Design review of the part built by this model. Coordinates are the model's own, in mm. A direction names the side the tool comes from. Coordinates: 2 decimals unless noted, no trailing zeros. Order: outer loops, then holes, each group sorted by start corner. A loop starts at its lowest first (then second) coordinate and runs counter-clockwise, first axis right, second up. Notation, with made-up numbers: (67.25, 60.25) - (106.25, 60.25) arc R30 ccw to (106.25, 96.25) - close; hole circle Ø5 at (-16.5, 39). An arc over 180 degrees is marked (long way). Write each question's results on one line, items separated by ' | '. Start each with the question number.
```python
from build123d import *

# Parameters (mm, degrees)
ESQUISSE1_R                  = 12.5
BOSS_EXTRU_1_DEPTH           = 34.6
BOSS_EXTRU_2_START           = -34.6
BOSS_EXTRU_2_DEPTH           = 34.6
R_P_TITION_CIRCULAIRE1_COUNT = 12
ESQUISSE5_R                  = 7.5
ENL_V_MAT_EXTRU_2_DEPTH      = 5
ESQUISSE6_R                  = 6
ENL_V_MAT_EXTRU_3_DEPTH      = 24.6
ENL_V_START                  = -5
ESQUISSE7_R                  = 7.5
ENL_V_MAT_EXTRU_4_DEPTH      = 5


with BuildPart() as part:
    # Esquisse1 → Boss.-Extru.1 (new body)
    with BuildSketch(Plane.XY):
        Circle(ESQUISSE1_R)
    extrude(amount=BOSS_EXTRU_1_DEPTH)

    # Esquisse3 → Boss.-Extru.2 (add)
    with BuildSketch(Plane.XY.offset(34.6).offset(BOSS_EXTRU_2_START)):
        with BuildLine():
            Line((-1, 17.810368556), (-2.169061089, 12.310368556))
            ThreePointArc((-2.169061089, 12.310368556), (0, 12.5), (2.169061089, 12.310368556))
            Line((2.169061089, 12.310368556), (1, 17.810368556))
            Line((1, 17.810368556), (-1, 17.810368556))
        make_face()
    boss_extru_2 = extrude(amount=BOSS_EXTRU_2_DEPTH)

    # R_p_tition circulaire1: Boss.-Extru.2 ×12 about axis
    r_p_tition_circulaire1_axis = Axis((0, 0, 0), (0, 0, 1))
    for i in range(1, R_P_TITION_CIRCULAIRE1_COUNT):
        add(boss_extru_2.rotate(r_p_tition_circulaire1_axis, i * 360 / R_P_TITION_CIRCULAIRE1_COUNT))

    # Esquisse5 → Enl_v. mat.-Extru.2 (cut)
    with BuildSketch(Plane.XY.offset(34.6)):
        Circle(ESQUISSE5_R)
    extrude(amount=-ENL_V_MAT_EXTRU_2_DEPTH, mode=Mode.SUBTRACT)

    # Esquisse6 → Enl_v. mat.-Extru.3 (cut)
    with BuildSketch(Plane.XY.offset(29.6)):
        Circle(ESQUISSE6_R)
    extrude(amount=-ENL_V_MAT_EXTRU_3_DEPTH, mode=Mode.SUBTRACT)

    # Esquisse7 → Enl_v. mat.-Extru.4 (cut)
    with BuildSketch(Plane(origin=(0, 0, 0), x_dir=(-1, 0, 0), z_dir=(0, 0, -1)).offset(ENL_V_START)):
        with Locations(Location((0, 0, 0), (0, 0, 180))):
            Circle(ESQUISSE7_R)
    extrude(amount=ENL_V_MAT_EXTRU_4_DEPTH, mode=Mode.SUBTRACT)


solid = part.part
```
(1) Take a section at D-D (x = 10.5). State the section outline as (y, z) points, plus the area to 3 significant figures.
(2) Take a section at C-C (x = -13). State the section outline as (y, z) points, plus the area to 3 significant figures.
(3) Tool access review of faces 1 (the face through (6.132, -13.806, 17.058)), 2 (the face through (-15.022, 1.593, 17.058)), 3 (the face through (3.25, 12.07, 17.06)), 4 (the face through (-8.85, -8.83, 17.06)): name each direction out of +Z, -Z, +X, -X, +Y, -Y from which nothing blocks a thin tool from reaching the whole face with its end or side.
(4) Clearance check with flat-ended pins moving along their axes: pin 1 (9 mm diameter, centred on x = 0, y = 0, fed in from -Z); pin 2 (1 mm diameter, centred on x = 8.5, z = 26.5, fed in from +Y); pin 3 (10 mm diameter, centred on y = 8.5, z = 9.5, fed in from +X); pin 4 (2 mm diameter, centred on x = 4, z = 14.5, fed in from -Y). State where each tip first meets the part, or that it passes through.
(5) Take a section at A-A (y = 0). State the section outline as (x, z) points.
(6) To check wall thickness, follow line 1 along Y through (x, z) = (0, 4); line 2 along Y through (x, z) = (14, 18); line 3 along Y through (x, z) = (0, 16.25). State the ranges of each line that lie inside material, in increasing order. Write a range as [from, to].
(7) Mouldability with a two-part tool opening along Y and no side actions: class faces 5 (the face through (15.431, 8.893, 17.058)), 6 (the face through (-17.81, 0, 17)), 7 (the face through (12.07, -3.25, 17.06)) as +Y half, -Y half, draft (parallel to the pull), parting line (faces both ways), or undercut.
Worked out:
1) outline: (-8.33, 0) - (8.33, 0) - (8.33, 34.6) - (-8.33, 34.6) - close | area: 577 mm^2
2) outline: (-9.15, 0) - (-5.41, 0) - (-5.41, 34.6) - (-9.15, 34.6) - close; (-2.02, 0) - (2.02, 0) - (2.02, 34.6) - (-2.02, 34.6) - close; (5.41, 0) - (9.15, 0) - (9.15, 34.6) - (5.41, 34.6) - close | area: 399 mm^2
3) face 1: +Z, -Z, -Y | face 2: +Z, -Z, -X | face 3: +Z, -Z, +Y | face 4: +Z, -Z
4) pin 1: through | pin 2: y = 15.92 | pin 3: x = 15.92 | pin 4: y = -12.55
5) outline: (-17.81, 0) - (-7.5, 0) - (-7.5, 5) - (-6, 5) - (-6, 29.6) - (-7.5, 29.6) - (-7.5, 34.6) - (-17.81, 34.6) - close; (6, 5) - (7.5, 5) - (7.5, 0) - (17.81, 0) - (17.81, 34.6) - (7.5, 34.6) - (7.5, 29.6) - (6, 29.6) - close
6) line 1: [-17.81, -7.5], [7.5, 17.81] | line 2: [-9.47, -6.31], [-1.81, 1.81], [6.31, 9.47] | line 3: [-17.81, -6], [6, 17.81]
7) face 5: +Y half | face 6: draft | face 7: undercut
